Work out the finished part from the listing and answer in its coordinate system (mm). Face numbers are marked on the shaded views. A direction names the side the tool comes from. Round coordinates to 2 decimals unless told otherwise and drop trailing zeros. Loops run counter-clockwise (first coordinate to the right, second up) from the corner with the lowest first, then second, coordinate; pieces in that order, holes last. Notation, with made-up numbers: (64.25, 6.5) -> (75.25, 6.5) arc R23 ccw to (75.25, 16.5) -> close; hole circle Ø6 at (-5.75, 34). An arc over 180 degrees is marked (long way). Use one line per item in the form item = value.
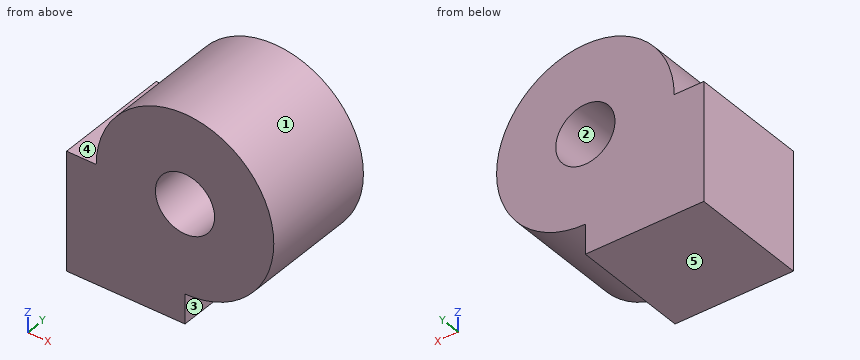
```python
from build123d import *

# Parameters (mm, degrees)
F1_DEPTH = 25.4
F2_R     = 6.35
F3_DEPTH = 25.4


with BuildPart() as f1:
    # F0 (on Front) → F1 (new body)
    with BuildSketch(Plane.XZ):
        with BuildLine():
            Line((0, 25.4), (0, 0))
            Line((0, 0), (25.4, 0))
            Line((25.4, 0), (25.4, 6.35))
            ThreePointArc((25.4, 6.35), (38.870384, 38.870384), (6.35, 25.4))
            Line((6.35, 25.4), (0, 25.4))
        make_face()
    extrude(amount=F1_DEPTH)

    # F2 (on face) → F3 (cut)
    with BuildSketch(Plane.XZ.offset(25.4)):
        with Locations((25.4, 25.4)):
            Circle(F2_R)
    extrude(amount=-F3_DEPTH, mode=Mode.SUBTRACT)


solid = f1.part
```
(1) For a pull along Z with two mould halves and no side action, classify the marked faces 1, 2 and 3 as +Z half, -Z half, draft (parallel to the pull), parting line (faces both ways), or undercut.
Completed:
face_1 = parting line
face_2 = undercut
face_3 = draft
(2) For the marked faces 4 and 5, determine the directions among +Z, -Z, +X, -X, +Y, -Y from which every point of the face is accessible in a straight line to the end or side of a thin tool.
Completed:
face_4 = +Z, -X, +Y, -Y
face_5 = -Z, +X, -X, +Y, -Y
(3) Consider L1, parallel to Z at x = 20, y = -10.75; L2, parallel to Z at x = 28.5, y = -8.75; L3, parallel to X at y = -20.5, z = 30.5. Determine where each line is inside the solid, lowest interval first.
Completed:
L1 = 0 to 22.06, 28.74 to 43.67
L2 = 6.6 to 19.86, 30.94 to 44.2
L3 = 7.05 to 21.62, 29.18 to 43.75
(4) Find section A-A, the plane z = 24. Write down the section's boundary in (x, y), then the cut area to 3 significant figures.
Completed:
outline = (0, -25.4) -> (19.21, -25.4) -> (19.21, 0) -> (0, 0) -> close; (31.59, -25.4) -> (44.4, -25.4) -> (44.4, 0) -> (31.59, 0) -> close
area = 813 mm2
(5) Find section C-C, the plane y = -19.5. Write down the section's boundary in (x, z), then the cut area to 3 significant figures.
Completed:
outline = (0, 0) -> (25.4, 0) -> (25.4, 6.35) arc R19.05 ccw (long way) to (6.35, 25.4) -> (0, 25.4) -> close; hole circle Ø12.7 at (25.4, 25.4)
area = 1,370 mm2
(6) Find section B-B, the plane x = 29.5. Write down the section's boundary in (y, z).
Completed:
outline = (-25.4, 6.8) -> (0, 6.8) -> (0, 20.55) -> (-25.4, 20.55) -> close; (-25.4, 30.25) -> (0, 30.25) -> (0, 44) -> (-25.4, 44) -> close
(7) Given P1, Ø3, axis at y = -12.5, z = 22.5, coming from the +X side; P2, Ø3, axis at y = -3, z = 39.5, coming from the +X side; P3, Ø10, axis at y = -7, z = 15, coming from the +X side, each flat-ended and moving along its own axis, determine where each tip first touches the part or whether it passes through.
Completed:
P1 = 44.4
P2 = 39.69
P3 = 43.67
(8) Find section D-D, the plane z = 12. Write down the section's boundary in (x, y), then the cut area to 3 significant figures.
Completed:
outline = (0, -25.4) -> (38.94, -25.4) -> (38.94, 0) -> (0, 0) -> close
area = 989 mm2
